Part model, mm, in its own coordinate system. A direction names the side the tool comes from. Coordinates: 2 decimals unless noted, no trailing zeros. Write each loop counter-clockwise with the first axis right and the second up, starting at its lowest first coordinate (ties: lowest second). Pieces come first, ordered by that corner, then holes. Notation, with made-up numbers: (49, 78) - (97, 78) arc R20 ccw to (97, 98) - close; hole circle Ø3 at (-32, 46). An arc over 180 degrees is marked (long way). Write each question's results on one line, items separated by ' | '.
from build123d import *

# Parameters (mm, degrees)
F0_W      = 50.8
F0_H      = 6.35
F1_DEPTH  = 2.54
F3_DEPTH  = 2.54
F6_DEPTH  = 3.81
F8_DEPTH  = 6.35
F9_R      = 1.9685
F10_DEPTH = 6.35


with BuildPart() as f1:
    # F0 (on Top) → F1 (new body)
    with BuildSketch(Plane.XY):
        with Locations((25.4, 0)):
            Rectangle(F0_W, F0_H)
    extrude(amount=F1_DEPTH)

    # F2 (on face) → F3 (cut)
    with BuildSketch(Plane.XY.offset(2.54)):
        with BuildLine():
            Line((50.8, -1.716926), (50.8, 1.716926))
            ThreePointArc((50.8, 1.716926), (49.083074, 0), (50.8, -1.716926))
        make_face()
    extrude(amount=-F3_DEPTH, mode=Mode.SUBTRACT)

    # F1_face (on face) → F4 (revolve)
    with BuildSketch(Plane(origin=(25.4, 0, 2.54), x_dir=(1, 0, 0), z_dir=(0, 0, 1))):
        with BuildLine():
            Line((25.4, 1.716926), (25.4, 3.175))
            Line((25.4, 3.175), (-25.4, 3.175))
            Line((-25.4, 3.175), (-25.4, -3.175))
            Line((-25.4, -3.175), (25.4, -3.175))
            Line((25.4, -3.175), (25.4, -1.716926))
            ThreePointArc((25.4, -1.716926), (23.683074, 0), (25.4, 1.716926))
        make_face()
    revolve(axis=Axis((0, 0, 2.54), (0, -1, 0)))

    # F5 (on face) → F6 (join)
    with BuildSketch(Plane(origin=(0, 3.175, 0), x_dir=(-1, 0, 0), z_dir=(0, 1, 0))):
        Polygon((5.865879, 10.16), (-5.865879, 10.16), (-11.731757, 0), (-5.865879, -10.16), (5.865879, -10.16), (11.731757, 0), align=None)
    extrude(amount=F6_DEPTH)

    # F7 (on face) → F8 (cut)
    with BuildSketch(Plane(origin=(0, 6.985, 0), x_dir=(-1, 0, 0), z_dir=(0, 1, 0))):
        Polygon((4.05375, 7.021301), (-4.05375, 7.021301), (-8.107501, 0), (-4.05375, -7.021301), (4.05375, -7.021301), (8.107501, 0), align=None)
    extrude(amount=-F8_DEPTH, mode=Mode.SUBTRACT)

    # F9 (on face) → F10 (cut)
    with BuildSketch(Plane(origin=(0, 0.635, 0), x_dir=(-1, 0, 0), z_dir=(0, 1, 0))):
        Circle(F9_R)
    extrude(amount=-F10_DEPTH, mode=Mode.SUBTRACT)


solid = f1.part
(1) 3-axis set-ups, long thin cutter, end or side, ignore diameter. For faces 1 (the flat face through (-8.84, 5.05, 5.01)), 2 (the flat face through (-2, 0.635, 2)), 3 (the flat face through (-8.76, 5.05, -5.15)), 4 (the flat face through (0, 5, -10.16)): which of +Z, -Z, +X, -X, +Y, -Y reach the whole face in a straight line?
Return value:
face 1: +Z, -X, +Y | face 2: +Y | face 3: -Z, -X, +Y | face 4: -Z, +X, -X, +Y
(2) Wall check: line 1 (Z direction, x = 0, y = -2.2); line 2 (Y direction, x = -15.5, z = 16.5) (3 decimals); line 3 (Z direction, x = 3, y = 1.25). Give the ranges that are in metal, low to high. Write a range as from..to.
Return value:
line 1: z = -48.26..-1.97, 1.97..53.34 | line 2: y = -3.175..3.175 | line 3: z = -46.99..-7.02, 7.02..52.07
(3) Two-plate mould, pull along Y, no slides. Class faces 5 (the flat face through (11, 3.175, 3)), 6 (the cylindrical face through (0.43, -1.24, -1.92)), 7 (the cylindrical face through (49.083, 0.038, 1.288)): released by +Y, released by -Y, zero draft, split by the parting line, or undercut.
Return value:
face 5: released by +Y | face 6: zero draft | face 7: undercut
(4) Saw through at A-A on x = 0. Write the cut outline in (y, z) (1 decimal), then the cut area to 3 significant figures.
Return value:
outline: (-3.2, -48.3) - (-1.7, -48.3) arc R1.7 cw to (1.7, -48.3) - (3.2, -48.3) - (3.2, -10.2) - (7, -10.2) - (7, -7) - (0.6, -7) - (0.6, -2) - (-3.2, -2) - close; (-3.2, 2) - (0.6, 2) - (0.6, 7) - (7, 7) - (7, 10.2) - (3.2, 10.2) - (3.2, 53.3) - (1.7, 53.3) arc R1.7 cw to (-1.7, 53.3) - (-3.2, 53.3) - close | area: 609 mm^2
(5) Flat gauge pins, fed straight in: P1, Ø3, axis at x = 0, z = 0, coming from the -Y side; P2, Ø1.9, axis at x = 1.5, y = 5, coming from the -Z side; P3, Ø8, axis at x = 24, z = 0.5, coming from the +Y side (3 decimals); P4, Ø1.1, axis at x = -0.5, y = 5.5, coming from the +Z side. Where does each tip first touch, or does it go through?
Return value:
P1: passes through | P2: stops at z = -10.16 | P3: stops at y = 3.175 | P4: stops at z = 10.16
